Drawing for the job (mm, zero at the part's lowest x, y, z). Give positions to 0.01 mm unless a question says otherwise; leave off trailing zeros. Write each loop counter-clockwise with the first axis right and the second up, starting at its lowest first coordinate (ties: lowest second). Pieces come first, ordered by that corner, then holes. Notation, with made-up numbers: (69.25, 15) - (85.25, 15) arc R17 cw to (85.25, 29) - close; hole circle Ø7 at (6.5, 51). An arc over 180 degrees is marked (long way). Write item = value, one per line. Start each with the question number.
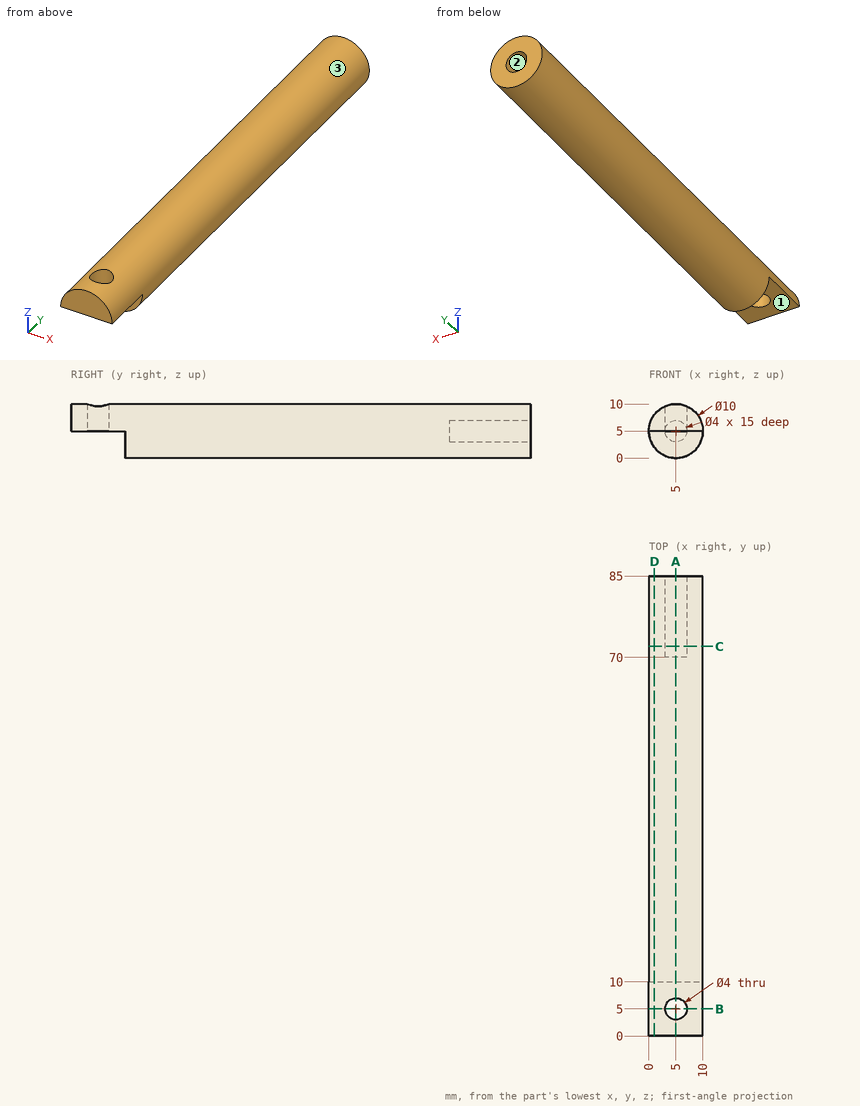
1. Wall check: line 1 along Z through (x, y) = (5, 78.75); line 2 along Y through (x, z) = (5, 6.9); line 3 along Y through (x, z) = (5, 8.35). Give the ranges that are in metal, low to high.
2. Cut at B-B (y = 5). Give the cut face in (x, z), then the cut area to 3 significant figures.
3. Cut at C-C (y = 72). Give the cut face in (x, z), then the cut area to 3 significant figures.
4. Pin check, flat tips, straight feed: pin 1 Ø6 at (x, y) = (8, 49.5) entering from +Z; pin 2 Ø1.5 at (x, z) = (4, 2) entering from -Y. Stop position of each tip, or through.
5. Cut at A-A (x = 5). Give the cut face in (y, z), then the cut area to 3 significant figures.
6. Cut at D-D (x = 1). Give the cut face in (y, z), then the cut area to 3 significant figures.
7. Mould opens along Z. For the marked faces 1, 2 and 3 say: +Z half, -Z half, draft (parallel to the pull), parting line (faces both ways), or undercut.
Output:
q1.line_1 = 0 to 3, 7 to 10
q1.line_2 = 0 to 3, 7 to 70
q1.line_3 = 0 to 3, 7 to 85
q2.outline = (0, 5) - (3, 5) - (3, 9.58) arc R5 ccw to start; (7, 5) - (10, 5) arc R5 ccw to (7, 9.58) - close
q2.area = 19.8 mm2
q3.outline = circle Ø10 at (5, 5); hole circle Ø4 at (5, 5)
q3.area = 66.0 mm2
q4.pin_1 = 10
q4.pin_2 = 10
q5.outline = (0, 5) - (3, 5) - (3, 10) - (0, 10) - close; (7, 5) - (10, 5) - (10, 0) - (85, 0) - (85, 3) - (70, 3) - (70, 7) - (85, 7) - (85, 10) - (7, 10) - close
q5.area = 720 mm2
q6.outline = (0, 5) - (10, 5) - (10, 2) - (85, 2) - (85, 8) - (0, 8) - close
q6.area = 480 mm2
q7.face_1 = -Z half
q7.face_2 = undercut
q7.face_3 = parting line
